from build123d import *

# Parameters (mm, degrees)
SKETCH1_W                = 2.54
SKETCH1_H                = 2.54
SKETCH1_W_2              = 0.68
SKETCH1_H_2              = 0.68
BOSS_EXTRUDE1_DEPTH      = 8.4
SKETCH2_W                = 1
SKETCH2_H                = 1
CUT_EXTRUDE1_DEPTH       = 7
CHAMFER1_SIZE            = 0.5
BOSS_EXTRUDE2_DEPTH      = 0.5
BOSS_EXTRUDE2_DEPTH_BACK = 0.5
SKETCH4_W                = 0.16
SKETCH4_H                = 6.500631374
BOSS_EXTRUDE3_DEPTH      = 3
BOSS_EXTRUDE3_DEPTH_BACK = 1
SKETCH7_W                = 0.68
SKETCH7_H                = 0.68
SKETCH8_W                = 1
SKETCH8_H                = 1
SKETCH8_W_2              = 0.68
SKETCH8_H_2              = 0.68
BOSS_EXTRUDE4_DEPTH      = 0.499368626
CHAMFER2_SIZE            = 0.2


with BuildPart() as part:
    # Sketch1 → Boss-Extrude1 (new body)
    with BuildSketch(Plane(origin=(0, 0, 0), x_dir=(1, 0, 0), z_dir=(0, 1, 0))):
        Rectangle(SKETCH1_W, SKETCH1_H)
        Rectangle(SKETCH1_W_2, SKETCH1_H_2, mode=Mode.SUBTRACT)
    extrude(amount=BOSS_EXTRUDE1_DEPTH)

    # Sketch2 → Cut-Extrude1 (cut)
    with BuildSketch(Plane(origin=(0, 8.4, 0), x_dir=(1, 0, 0), z_dir=(0, 1, 0))):
        Rectangle(SKETCH2_W, SKETCH2_H)
    extrude(amount=-CUT_EXTRUDE1_DEPTH, mode=Mode.SUBTRACT)

    # Chamfer1
    chamfer1_edges = [part.edges().sort_by_distance(p)[0] for p in [
        (0.34, 0, 0),
        (0, 0, -0.34),
        (-0.34, 0, 0),
        (0, 0, 0.34),
    ]]
    chamfer(chamfer1_edges, length=CHAMFER1_SIZE)

    # Sketch4 → Boss-Extrude2 (add, two sides: drawn at the far end of the back side and taken through both)
    with BuildSketch(Plane.XY.offset(-BOSS_EXTRUDE2_DEPTH_BACK)):
        with Locations((-0.42, 4.650315687)):
            Rectangle(SKETCH4_W, SKETCH4_H)
        with Locations((0.42, 4.650315687)):
            Rectangle(SKETCH4_W, SKETCH4_H)
    extrude(amount=BOSS_EXTRUDE2_DEPTH + BOSS_EXTRUDE2_DEPTH_BACK)

    # Sketch7 → Boss-Extrude3 (add, two sides: drawn at the far end of the back side and taken through both)
    with BuildSketch(Plane(origin=(0, 7.900631374, 0), x_dir=(1, 0, 0), z_dir=(0, 1, 0)).offset(-BOSS_EXTRUDE3_DEPTH_BACK)):
        Rectangle(SKETCH7_W, SKETCH7_H)
    extrude(amount=BOSS_EXTRUDE3_DEPTH + BOSS_EXTRUDE3_DEPTH_BACK)

    # Sketch8 → Boss-Extrude4 (add)
    with BuildSketch(Plane(origin=(0, 8.4, 0), x_dir=(1, 0, 0), z_dir=(0, 1, 0))):
        Rectangle(SKETCH8_W, SKETCH8_H)
        Rectangle(SKETCH8_W_2, SKETCH8_H_2, mode=Mode.SUBTRACT)
    extrude(amount=-BOSS_EXTRUDE4_DEPTH)

    # Chamfer2
    chamfer2_edges = [part.edges().sort_by_distance(p)[0] for p in [
        (0.34, 10.900631374, 0),
        (0, 10.900631374, -0.34),
        (-0.34, 10.900631374, 0),
        (0, 10.900631374, 0.34),
    ]]
    chamfer(chamfer2_edges, length=CHAMFER2_SIZE)


solid = part.part
Here's how the part is built. I have some questions about the finished solid (model axes, mm). A direction names the side the tool comes from. Round coordinates to 2 decimals unless told otherwise and drop trailing zeros. Loops run counter-clockwise (first coordinate to the right, second up) from the corner with the lowest first, then second, coordinate; pieces in that order, holes last. Notation, with made-up numbers: M 24.5,-35.75 L 82.5,-35.75 A16 cw 82.5,-31.75 Z; hole C 72.5,58 d5. An arc over 180 degrees is marked long. Write each question's results on one line, items separated by ' | '. Start each with the question number.
(1) I want a section at A-A (x = 0.45). Please give me the cut outline in (y, z).
(2) I want a section at B-B (y = 0.75). Please give me the cut outline in (x, z), then the cut area to 3 significant figures.
(3) I want a section at D-D (y = 3). Please give me the cut outline in (x, z), then the cut area to 3 significant figures.
(4) I want a section at C-C (z = 0.6). Please give me the cut outline in (x, y).
(5) On a 3-axis mill with a long thin cutter (end or side, diameter ignored), from which of +Z, -Z, +X, -X, +Y, -Y can I reach the whole of each face in a straight line? I mean faces 1 (the flat face through (-0.34, 4, 0)), 2 (the flat face through (0, 4, 1.27)), 3 (the flat face through (1, 8.4, 0)). Say none if no direction works.
(6) Thinking about a two-plate mould opening in X: for faces 4 (the flat face through (0.34, 4, 0)), 5 (the flat face through (0, 4, -1.27)), 6 (the flat face through (-1.27, 4, 0)), which applies, pulls with the +X half, pulls with the -X half, needs draft (parallel to the pull), parting line crosses it, or undercut?
(7) If I drill on probe 1 along Z at (x, y) = (0.3, 4.25); probe 2 along X at (y, z) = (5, -0.2); probe 3 along Y at (x, z) = (-1.1, -1.05), over which ranges is the centre line in solid material (lowest first)? Write a range as from..to.
(8) Will these pins go through, and if not, where does the flat tip stop? P1, Ø0.7, axis at y = 9.5, z = 0, coming from the +X side; P2, Ø0.5, axis at x = 0, z = 0, coming from the -Y side.
Solved:
1) outline: M 0,-1.27 L 8.4,-1.27 L 8.4,1.27 L 0,1.27 L 0,0.84 L 0.39,0.45 L 0.39,-0.45 L 0,-0.84 Z
2) outline: M -1.27,-1.27 L 1.27,-1.27 L 1.27,1.27 L -1.27,1.27 Z; hole M -0.34,-0.34 L 0.34,-0.34 L 0.34,0.34 L -0.34,0.34 Z | area: 5.99 mm²
3) outline: M -1.27,-1.27 L 1.27,-1.27 L 1.27,1.27 L -1.27,1.27 Z; hole M -0.34,-0.5 L 0.34,-0.5 L 0.34,0.5 L -0.34,0.5 Z | area: 5.77 mm²
4) outline: M -1.27,0 L -0.84,0 L -0.6,0.24 L 0.6,0.24 L 0.84,0 L 1.27,0 L 1.27,8.4 L -1.27,8.4 Z
5) face 1: none | face 2: +Z, +X, -X, +Y, -Y | face 3: +Y
6) face 4: undercut | face 5: needs draft | face 6: pulls with the -X half
7) probe 1: z = -1.27..-0.5, 0.5..1.27 | probe 2: x = -1.27..-0.34, 0.34..1.27 | probe 3: y = 0..8.4
8) P1: stops at x = 0.34 | P2: stops at y = 6.9
